```python
from build123d import *

# Parameters (mm, degrees)
FILLET002_R        = 1.49
FILLET003_R        = 2
SKETCH006_W        = 7.538901
SKETCH006_H        = 2
POCKET_DEPTH       = 3
POLARPATTERN_COUNT = 6
FILLET017_R        = 1.49


with BuildPart() as part:
    # Sketch001 → Revolution001 (revolve)
    with BuildSketch(Plane.XZ):
        Polygon((0, 5), (5, 5), (5, 0), (12.5, 0), (12.5, 2), (11.5, 3), (12.5, 4), (12.5, 6), (9.224268, 15), (11.224268, 15), (11.224268, 18), (8.198129, 18), (5.675519, 31.680297), (8, 35), (8, 43), (6, 43), (6, 40), (0, 40), align=None)
    revolve(axis=Axis((0, 0, 0), (0, 0, 1)))

    # Fillet002
    fillet002_edges = [part.edges().sort_by_distance(p)[0] for p in [
        (12, 0, 3.5),
        (-12.5, 0, 4),
    ]]
    fillet(fillet002_edges, radius=FILLET002_R)

    # Fillet003
    fillet003_edges = [part.edges().sort_by_distance(p)[0] for p in [
        (-6, 0, 40),
    ]]
    fillet(fillet003_edges, radius=FILLET003_R)

    # Sketch006 → Pocket (cut)
    with BuildSketch(Plane(origin=(0, 0, 43), x_dir=(-1, 0, 0), z_dir=(0, 0, 1))):
        with Locations((9.347359, 0)):
            Rectangle(SKETCH006_W, SKETCH006_H)
    pocket = extrude(amount=-POCKET_DEPTH, mode=Mode.SUBTRACT)

    # PolarPattern: Pocket ×6 about axis
    polarpattern_axis = Axis((0, 0, 43), (0, 0, 1))
    for i in range(1, POLARPATTERN_COUNT):
        add(pocket.rotate(polarpattern_axis, i * 360 / POLARPATTERN_COUNT), mode=Mode.SUBTRACT)

    # Fillet017
    fillet017_edges = [part.edges().sort_by_distance(p)[0] for p in [
        (-11.224268, 0, 18),
        (-11.224268, 0, 15),
    ]]
    fillet(fillet017_edges, radius=FILLET017_R)


solid = part.part
```
Geometry: final body of the model. Coordinates: model frame, mm. A direction names the side the tool comes from. Coordinates: 2 decimals unless noted, no trailing zeros. Order: outer loops, then holes, each group sorted by start corner. A loop starts at its lowest first (then second) coordinate and runs counter-clockwise, first axis right, second up.
Item 1: Contact query for flat-ended pins moving along their axis: P1, Ø8, axis at x = 0, y = 0, coming from the -Z side; P2, Ø0.7, axis at x = 7, z = 41.5, coming from the +Y side; P3, Ø2, axis at y = -7, z = 17, coming from the -X side. Output: stop coordinate, or through.
Answer:
P1: stops at z = 5
P2: stops at y = 4.45
P3: stops at x = -9.44
Item 2: Access query for faces 1 (the face through (-2.777, 4.838, 40.454)), 2 (the face through (-1.08, -4.88, 2.46)), 3 (the face through (7, 1, 42)), 4 (the face through (-7, -1, 42)). Directions: +Z, -Z, +X, -X, +Y, -Y. A direction counts if a zero-diameter tool reaches every point of the face in a straight line with its end or side. Return the directions, or none.
Answer:
face 1: +Z
face 2: -Z
face 3: +Z, +X
face 4: +Z, -X
Item 3: Section query A-A (z = 31). Output: boundary loops of the cut face in (x, y).
Answer:
outline: circle Ø11.6 at (0, 0)
Item 4: Material intervals for line 1 along Y through (x, z) = (0, 1.1); line 2 along Z through (x, y) = (-7.25, 4.75); line 3 along Z through (x, y) = (-6.75, -9.5), sorted ascending.
Answer:
line 1: y = -12.5 to -5, 5 to 12.5
line 2: z = 0 to 18
line 3: z = 0 to 2.85, 3.15 to 8.32
Item 5: Draft query along Z for faces 5 (the face through (-2.113, -9.516, 13.563)), 6 (the face through (6, -4, 43)), 7 (the face through (-5.211, -2.974, 42.493)). Return one class per face: released by +Z, released by -Z, zero draft, split by the parting line, or undercut.
Answer:
face 5: undercut
face 6: released by +Z
face 7: zero draft
